Part model, mm, in its own coordinate system. A direction names the side the tool comes from. Round coordinates to 2 decimals unless told otherwise and drop trailing zeros. Order: outer loops, then holes, each group sorted by start corner. A loop starts at its lowest first (then second) coordinate and runs counter-clockwise, first axis right, second up. Notation, with made-up numbers: (-9, 24) -> (32, 24) arc R8 ccw to (32, 39) -> close; hole circle Ø11 at (47.5, 54). An arc over 180 degrees is marked (long way). Answer as a JSON object with one key per item and string values. Group by question number.
```python
from build123d import *
from OCP.BRepFilletAPI import BRepFilletAPI_MakeChamfer

# Parameters (mm, degrees)
SKETCH1_W           = 82.55
SKETCH1_H           = 25.4
SKETCH1_R           = 2.54
BOSS_EXTRUDE1_DEPTH = 25.4
CHAMFER1_SIZE       = 15.24
CHAMFER1_SIZE2      = 35.903190055
FILLET1_R           = 10
CHAMFER2_SIZE       = 5.08
CHAMFER2_SIZE_2     = 145.472166677
BOSS_EXTRUDE2_DEPTH = 25.4
SKETCH3_R           = 2.54
CUT_EXTRUDE1_DEPTH  = 92.63619095
SKETCH4_R           = 2.54
CUT_EXTRUDE2_DEPTH  = 92.63619095
FILLET3_R           = 7.62
FILLET4_R           = 7.62
SKETCH5_R           = 6.35
SKETCH5_R_2         = 2.54
BOSS_EXTRUDE3_DEPTH = 25.4
FILLET5_R           = 7.62
CUT_EXTRUDE3_DEPTH  = 91.009898604
FILLET6_R           = 7.62


with BuildPart() as part:
    # Sketch1 → Boss-Extrude1 (new body)
    with BuildSketch(Plane(origin=(0, 0, 0), x_dir=(1, 0, 0), z_dir=(0, 1, 0))):
        with Locations((32.385, 3.81)):
            Rectangle(SKETCH1_W, SKETCH1_H)
        with Locations(Location((0, 0, 0), (0, 0, 270))):
            Circle(SKETCH1_R, mode=Mode.SUBTRACT)
    extrude(amount=BOSS_EXTRUDE1_DEPTH)

    # Chamfer1: one chamfer whose edges measure the first distance from different faces: ONE call of the kernel's chamfer builder (chamfer() names one face for all edges)
    chamfer1_edges_1 = [part.edges().sort_by_distance(p)[0] for p in [
        (-8.89, 12.7, -16.51),
    ]]
    chamfer1_side_1 = [part.faces().sort_by_distance(p)[0] for p in [
        (-8.89, 12.7, -3.81),
    ]]
    chamfer1_edges_2 = [part.edges().sort_by_distance(p)[0] for p in [
        (73.66, 12.7, 8.89),
    ]]
    chamfer1_side_2 = [part.faces().sort_by_distance(p)[0] for p in [
        (73.66, 12.7, -3.81),
    ]]
    chamfer1 = BRepFilletAPI_MakeChamfer(part.part.solid().wrapped)
    for e in chamfer1_edges_1:
        chamfer1.Add(CHAMFER1_SIZE, CHAMFER1_SIZE2, e.wrapped, chamfer1_side_1[0].wrapped)  # the first distance lies on this face
    for e in chamfer1_edges_2:
        chamfer1.Add(CHAMFER1_SIZE, CHAMFER1_SIZE2, e.wrapped, chamfer1_side_2[0].wrapped)  # the first distance lies on this face
    add(Compound.cast(chamfer1.Shape()), mode=Mode.REPLACE)

    # Fillet1
    fillet1_edges = [part.edges().sort_by_distance(p)[0] for p in [
        (73.66, 12.7, -6.35),
    ]]
    fillet(fillet1_edges, radius=FILLET1_R)

    # Chamfer2
    # the kernel refuses this chamfer: 145.472166677, 5.08 mm, written as the material it takes off along each edge
    with BuildSketch(Plane(origin=(73.66, -378.219112331, -16.51), x_dir=(0.7401679873250444, 0, 0.6724220033127953), z_dir=(0, 1, 0))) as chamfer2_piece_1:
        Polygon((CHAMFER2_SIZE * 0.672422003313, -CHAMFER2_SIZE * 0.740167987325), (-CHAMFER2_SIZE_2 * 0.740167987326, -CHAMFER2_SIZE_2 * 0.672422003314), (0, 0), align=None)
    extrude(amount=781.838224662, mode=Mode.SUBTRACT)

    # Sketch2 → Boss-Extrude2 (add)
    with BuildSketch(Plane(origin=(0, 25.4, 0), x_dir=(1, 0, 0), z_dir=(0, 1, 0))):
        Polygon((-3.433319289, 3.586223542), (-44.714941303, -35.935291914), (-32.770661076, -48.411515456), (8.510960938, -8.89), align=None)
    extrude(amount=-BOSS_EXTRUDE2_DEPTH)

    # Sketch3 → Cut-Extrude1 (cut, through all)
    with BuildSketch(Plane(origin=(0, 25.4, 0), x_dir=(1, 0, 0), z_dir=(0, 1, 0))):
        with Locations(Location((0, 0, 0), (0, 0, 270))):
            Circle(SKETCH3_R)
    extrude(amount=-CUT_EXTRUDE1_DEPTH, mode=Mode.SUBTRACT)

    # Sketch4 → Cut-Extrude2 (cut, through all)
    with BuildSketch(Plane(origin=(0, 25.4, 0), x_dir=(1, 0, 0), z_dir=(0, 1, 0))):
        with Locations(Location((-34.808399123, -37.000207438, 0), (0, 0, 270))):
            Circle(SKETCH4_R)
    extrude(amount=-CUT_EXTRUDE2_DEPTH, mode=Mode.SUBTRACT)

    # Fillet3
    fillet3_edges = [part.edges().sort_by_distance(p)[0] for p in [
        (-44.714941303, 12.7, 35.935291914),
        (-32.770661076, 12.7, 48.411515456),
    ]]
    fillet(fillet3_edges, radius=FILLET3_R)

    # Fillet4
    fillet4_edges = [part.edges().sort_by_distance(p)[0] for p in [
        (37.756809945, 12.7, 8.89),
        (8.510960938, 12.7, 8.89),
    ]]
    fillet(fillet4_edges, radius=FILLET4_R)

    # Sketch5 → Boss-Extrude3 (add)
    with BuildSketch(Plane(origin=(0, 25.4, 0), x_dir=(1, 0, 0), z_dir=(0, 1, 0))):
        Circle(SKETCH5_R)
        with Locations(Location((0, 0, 0), (0, 0, 270))):
            Circle(SKETCH5_R_2, mode=Mode.SUBTRACT)
    extrude(amount=-BOSS_EXTRUDE3_DEPTH)

    # Fillet5
    fillet5_edges = [part.edges().sort_by_distance(p)[0] for p in [
        (2.173832351, 12.7, -5.966318204),
    ]]
    fillet(fillet5_edges, radius=FILLET5_R)

    # Sketch6 → Cut-Extrude3 (cut, through all)
    with BuildSketch(Plane(origin=(0, 25.4, 0), x_dir=(1, 0, 0), z_dir=(0, 1, 0))):
        Polygon((-5.801880984, 2.580828752), (-8.89, -1.637803048), (-8.89, 1.27), align=None)
    extrude(amount=-CUT_EXTRUDE3_DEPTH, mode=Mode.SUBTRACT)

    # Fillet6
    fillet6_edges = [part.edges().sort_by_distance(p)[0] for p in [
        (-5.801880984, 12.7, -2.580828752),
        (-8.89, 12.7, 1.637803048),
    ]]
    fillet(fillet6_edges, radius=FILLET6_R)


solid = part.part
```
Q1. Band-saw the part on A-A (z = 0). List the corners of the cut face in (x, y).
Q2. Drop flat-ended pins along their axis: pin 1 Ø4 at (y, z) = (19, 16.5) entering from -X; pin 2 Ø10 at (y, z) = (16, -1) entering from -X; pin 3 Ø7.5 at (x, y) = (21.5, 18.5) entering from +Z; pin 4 Ø1.5 at (x, z) = (22.5, -2) entering from -Y. Give the stop position or say it passes through.
Q3. Wall check: line 1 (X direction, y = 20.25, z = 36); line 2 (Z direction, x = -36, y = 7); line 3 (Z direction, x = 1, y = 3). Give the ranges that are in metal, low to high. Write a range as [from, to].
Q4. Band-saw the part on C-C (x = 62). List the corners of the cut face in (y, z).
Q5. Band-saw the part on D-D (z = 28). List the corners of the cut face in (x, y), plus the area to 3 significant figures.
Q6. Which spindle directions (+Z, -Z, +X, -X, +Y, -Y) get a long thin tool onto all of the face, cutting with end or side? Do faces 1 (the cylindrical face through (-41.56, 12.52, 36.09)), 2 (the flat face through (24, 13, 8.89)). Say none if no direction does.
Q7. Band-saw the part on B-B (y = 6). List the corners of the cut face in (x, z).
Completed:
{
 "1": {"outline": "(-7.69, 0) -> (-2.54, 0) -> (-2.54, 25.4) -> (-7.69, 25.4) -> close; (2.54, 0) -> (58.7, 0) -> (58.7, 25.4) -> (2.54, 25.4) -> close"},
 "2": {"pin 1": "x = -26.5", "pin 2": "x = -11.36", "pin 3": "z = 8.89", "pin 4": "y = 0"},
 "3": {"line 1": "[-41.56, -37.14], [-32.47, -19.81]", "line 2": "[27.59, 34.76], [39.24, 44.42]", "line 3": "[-6.29, -2.33], [2.33, 16.08]"},
 "4": {"outline": "(0, -11.84) -> (25.4, -11.84) -> (25.4, -1.4) -> (0, -1.4) -> close"},
 "5": {"outline": "(-36.43, 0) -> (-11.45, 0) -> (-11.45, 25.4) -> (-36.43, 25.4) -> close", "area": "634 mm2"},
 "6": {"face 1": "-X, +Y, -Y", "face 2": "+Z, +X, +Y, -Y"},
 "7": {"outline": "(-39.45, 41.44) arc R7.62 ccw to (-39.21, 30.67) -> (-9.37, 2.1) arc R7.62 cw to (-8.49, 1.1) -> (-6.19, -2.05) arc R7.62 cw to (-5.61, -2.98) arc R6.35 ccw to (0.62, -6.32) arc R7.62 cw to (4.35, -6.89) -> (19.5, -13.32) -> (73.54, -11.43) arc R10 ccw to (67.57, -3.76) -> (39.18, 8.28) arc R7.62 ccw to (36.21, 8.89) -> (11.57, 8.89) arc R7.62 cw to (6.3, 11.01) -> (-27.27, 43.14) arc R7.62 ccw to (-38.04, 42.91) -> close; hole circle Ø5.08 at (-34.81, 37); hole circle Ø5.08 at (0, 0)"}
}
